Print and shaded views of the part. All mm, measured from the part's lowest x, y and z. Coordinates: 2 decimals unless noted, no trailing zeros. Loops run counter-clockwise (first coordinate to the right, second up) from the corner with the lowest first, then second, coordinate; pieces in that order, holes last.
1) Pin check, flat tips, straight feed: pin 1 Ø12 at (x, z) = (28, 12) entering from -Y; pin 2 Ø8 at (x, y) = (6.5, 5) entering from -Z (1 decimal); pin 3 Ø1.5 at (x, y) = (55, 2) entering from +Z; pin 4 Ø4 at (y, z) = (7.5, 19) entering from +X (1 decimal). Stop position of each tip, or through.
2) Wall check: line 1 along Z through (x, y) = (32.5, 5.75) (1 decimal); line 2 along X through (y, z) = (12.5, 12.5) (1 decimal); line 3 along Z through (x, y) = (33, 2.75) (1 decimal). Give the ranges that are in metal, low to high.
3) Saw through at A-A, the plane x = 32.5. Write the cut outline in (y, z) (1 decimal).
4) Two-plate mould, pull along X, no slides. Class the marked faces 1, 2 and 3: +X half, -X half, draft (parallel to the pull), parting line (faces both ways), or undercut.
5) Saw through at D-D, the plane z = 45. Write the cut outline in (x, y), and give its area (3 significant figures).
6) Saw through at C-C, the plane x = 8.5. Write the cut outline in (y, z).
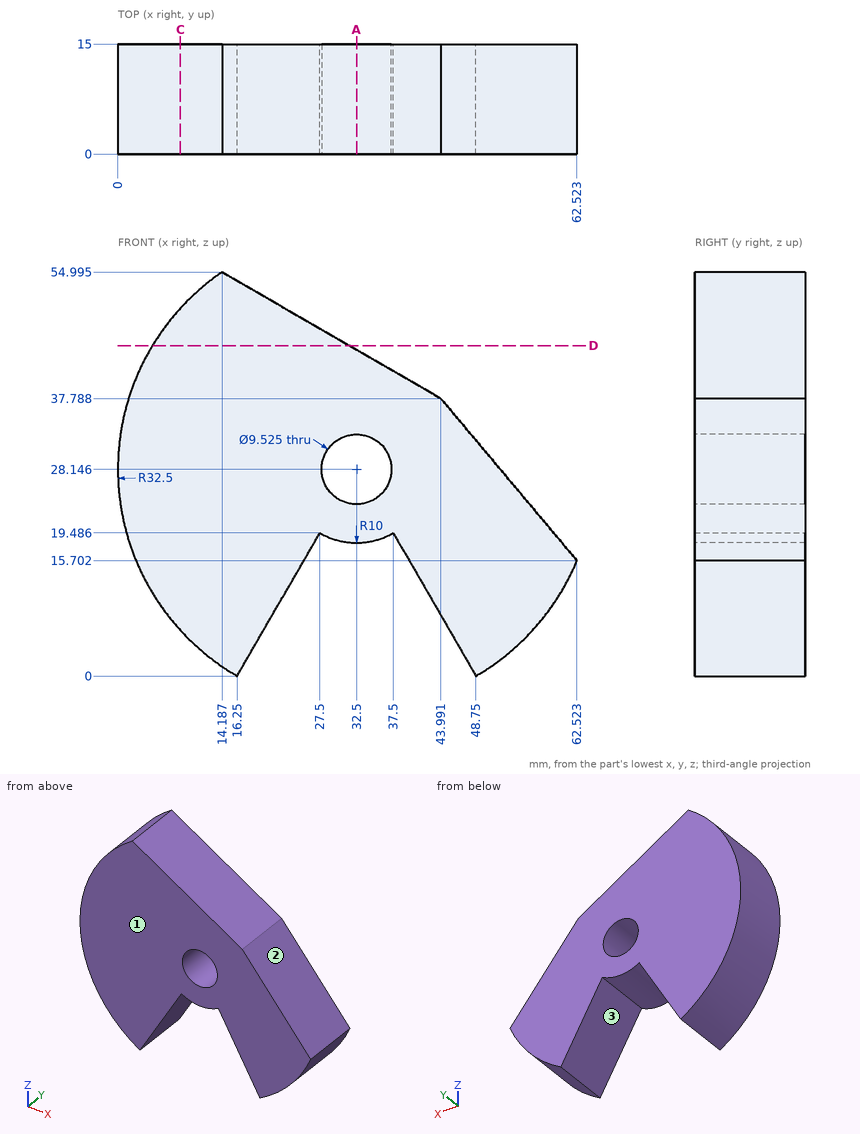
Data:
1. pin 1: stops at y = 0
1. pin 2: stops at z = 4.2
1. pin 3: stops at z = 25.56
1. pin 4: stops at x = 61.4
2. line 1: z = 18.1 to 23.4, 32.9 to 44.4
2. line 2: x = 4 to 23.5, 41.5 to 61
2. line 3: z = 18.2 to 23.4, 32.9 to 44.1
3. outline: (0, 18.1) - (15, 18.1) - (15, 23.4) - (0, 23.4) - close; (0, 32.9) - (15, 32.9) - (15, 44.4) - (0, 44.4) - close
4. face 1: draft
4. face 2: +X half
4. face 3: undercut
5. outline: (4.71, 0) - (31.5, 0) - (31.5, 15) - (4.71, 15) - close
5. area: 402 mm2
6. outline: (0, 6.23) - (15, 6.23) - (15, 50.06) - (0, 50.06) - close
